Could you check a few things on this model? Use its own coordinates, in mm. Round coordinates to 2 decimals unless told otherwise and drop trailing zeros. Use one line per item in the form item = value.
Autodesk Inventor part; units mm, degrees
ref_plane "YZ Plane" through (0, 0, 0) normal (1, 0, 0) x (0, 1, 0)
ref_plane "XZ Plane" through (0, 0, 0) normal (0, 1, 0) x (-1, 0, 0)
ref_plane "XY Plane" through (0, 0, 0) normal (0, 0, 1) x (1, 0, 0)
sketch "Sketch1" plane through (0, 0, 0) normal (0, 1, 0) x (-1, 0, 0)
  circle A0 centre (0, 0) radius 19
  circle A1 centre (0, 0) radius 14
  dimension "d0" = 38
  dimension "d1" = 28
extrude "Extrusion1" add sketch "Sketch1" along normal blind 25
sketch "Sketch2" plane through (0, 25, 0) normal (0, 1, 0) x (1, 0, 0)
  circle A0 centre (0, -16.5) radius 1.5
  circle A1 centre (0, 0) radius 14
  dimension "d4" = 3
  dimension "d5" = 16.5
extrude "Extrusion2" cut sketch "Sketch2" against normal blind 25 contours A0
pattern_circular "Circular Pattern1" count 24 over 360 about axis through (0, -10, 0) along (0, 1, 0) of "Extrusion2"
sketch "Sketch3" plane through (0, 0, 0) normal (0, 1, 0) x (-1, 0, 0)
  circle A0 centre (0, 0) radius 14
  circle A1 centre (0, 0) radius 13
  dimension "d11" = 26
extrude "Extrusion3" add sketch "Sketch3" along normal blind 10
chamfer "Chamfer1" distance 1 angle 45 1 edges at (13, 10, 0)
properties part number "Kolo"
Item 1: I need wall thicknesses on L1, parallel to Z at x = 0, y = 7; L2, parallel to X at y = 21.25, z = -9.5; L3, parallel to X at y = 21.75, z = -11.5. Which ranges of each line are inside material? Lowest first, please.
Found:
L1 = -19 to -18, -15 to -13, 13 to 15, 18 to 19
L2 = -16.45 to -15.12, -13.46 to -10.28, 10.28 to 13.46, 15.12 to 16.45
L3 = -15.12 to -13.16, -10.18 to -7.98, 7.98 to 10.18, 13.16 to 15.12
Item 2: Imagine slicing it at A-A on z = 0. State how many separate pieces and enclosed holes the cut face has, plus the area to 3 significant figures.
Found:
separate_pieces = 4
enclosed_holes = 0
area = 119 mm2
Item 3: If we mould it in two halves opening along Z, with no side actions, what happens to faces 1 (the face through (0.1, 25, 14.2)), 2 (the face through (-12.932, 17.395, 5.362))? For each: released by +Z, released by -Z, zero draft, split by the parting line, or undercut.
Found:
face_1 = zero draft
face_2 = undercut
Item 4: Will these pins go through, and if not, where does the flat tip stop? P1, Ø12, axis at x = -3.5, z = 4.5, coming from the -Y side; P2, Ø10, axis at x = -12, y = 3, coming from the +Z side; P3, Ø1.5, axis at y = 6.5, z = 2, coming from the +X side; P4, Ø12, axis at x = -3, y = 6.5, coming from the -Z side.
Found:
P1 = through
P2 = 17.66
P3 = 18.96
P4 = -19
